Geometry check sheet. Reference: the model listing, model coordinates, mm. A direction names the side the tool comes from. Round coordinates to 2 decimals unless told otherwise and drop trailing zeros. Order: outer loops, then holes, each group sorted by start corner. A loop starts at its lowest first (then second) coordinate and runs counter-clockwise, first axis right, second up. Notation, with made-up numbers: (64, 58.25) - (99, 58.25) arc R9 cw to (99, 67.25) - close; hole circle Ø6 at (57, 19.25). An arc over 180 degrees is marked (long way). Return JSON: item names as keys, results as strings. Group by question number.
Q1. Tool access check on faces 1 (the flat face through (0, 18, 35)), 2 (the flat face through (0, 17, 415)). Record the directions out of +Z, -Z, +X, -X, +Y, -Y that give a thin tool (end or side, any length) a straight path to the whole face; none if there is none.
Q2. Sectioned sample at B-B, the plane x = 15.5. Record the cut outline in (y, z), then the cut area to 3 significant figures.
Q3. Material ranges on line 1 along X through (y, z) = (-2.5, 481); line 2 along Y through (x, z) = (18, 464), recorded low to high.
Q4. Gauge pin test, flat end, axial feed: pin 1 Ø12 at (x, y) = (-23.5, 2) entering from +Z. Record the tip position at first contact, or that the pin passes through.
Q5. Sectioned sample at C-C, the plane z = 272. Record the cut outline in (x, y).
Q6. Sectioned sample at A-A, the plane y = 7. Record the cut outline in (x, z).
Q7. Draft check along X on faces 3 (the flat face through (0, 18, 805)), 4 (the flat face through (0, -17, 414)), 5 (the flat face through (27, 0, 414)), 6 (the flat face through (-30, 0, 414)). Enter one of: pulls with the +X half, pulls with the -X half, needs draft (parallel to the pull), parting line crosses it, or undercut.
```python
from build123d import *

# Parameters (mm, degrees)
F0_W     = 60
F0_H     = 40
F0_W_2   = 54
F0_H_2   = 34
F1_DEPTH = 840
F3_DEPTH = 60
F4_DEPTH = 60


with BuildPart() as f1:
    # F0 (on Top) → F1 (new body)
    with BuildSketch(Plane.XY):
        Rectangle(F0_W, F0_H)
        Rectangle(F0_W_2, F0_H_2, mode=Mode.SUBTRACT)
    extrude(amount=F1_DEPTH)

    # F2 (on face) → F3 (cut)
    with BuildSketch(Plane.YZ.offset(30)):
        Polygon((20, 840), (-17, 840), (20, 803), align=None)
        Polygon((-17, 0), (20, 0), (20, 37), align=None)
    extrude(amount=-F3_DEPTH, mode=Mode.SUBTRACT)

    # F2 (on face) → F4 (cut)
    with BuildSketch(Plane.YZ.offset(30)):
        Polygon((20, 0), (20, 37), (-17, 0), align=None)
    extrude(amount=-F4_DEPTH, mode=Mode.SUBTRACT)


solid = f1.part
```
Reply:
{
 "1": {"face 1": "-Z, +X, -X, +Y", "face 2": "+Z, -Z"},
 "2": {"outline": "(-20, 0) - (-17, 0) - (-17, 840) - (-20, 840) - close; (17, 34) - (20, 37) - (20, 803) - (17, 806) - close", "area": "4,830 mm^2"},
 "3": {"line 1": "-30 to -27, 27 to 30", "line 2": "-20 to -17, 17 to 20"},
 "4": {"pin 1": "z = 825.87"},
 "5": {"outline": "(-30, -20) - (30, -20) - (30, 20) - (-30, 20) - close; hole (-27, -17) - (27, -17) - (27, 17) - (-27, 17) - close"},
 "6": {"outline": "(-30, 24) - (-27, 24) - (-27, 816) - (-30, 816) - close; (27, 24) - (30, 24) - (30, 816) - (27, 816) - close"},
 "7": {"face 3": "needs draft", "face 4": "undercut", "face 5": "undercut", "face 6": "pulls with the -X half"}
}
